For this review, take the finished solid that the model builds, in its own axes (mm). Face numbers are marked on the shaded views. A direction names the side the tool comes from. Round coordinates to 2 decimals unless told otherwise and drop trailing zeros. Order: outer loops, then holes, each group sorted by start corner. A loop starts at its lowest first (then second) coordinate and runs counter-clockwise, first axis right, second up. Notation, with made-up numbers: M 34.25,79 L 48.25,79 A19 ccw 48.25,98 Z; hole C -7.5,12.25 d4. An arc over 180 degrees is marked long. Answer as a JSON object with one key per item and string values.
Autodesk Inventor part; units mm, degrees
ref_plane "bolt_XY" through (0, 0, 0) normal (1, 0, 0) x (0, 0, -1)
ref_plane "bolt_YZ" through (0, 0, 0) normal (0, 0, -1) x (0, 1, 0)
ref_plane "bolt_ZX" through (0, 0, 0) normal (0, 1, 0) x (1, 0, 0)
sketch "Sketch_1" plane through (0, 0, 0) normal (0, 0, 1) x (1, 0, 0)
  line L0 (10, 0) -> (-5, 0)
  line L1 (-5, 0) -> (-5, 4.25)
  line L2 (-5, 4.25) -> (0, 4.25)
  line L3 (0, 4.25) -> (0, 2.5)
  line L4 (0, 2.5) -> (9.5095, 2.5)
  line L5 (9.5095, 2.5) -> (10, 2.0095)
  line L6 (10, 2.0095) -> (10, 0)
  line L7 (10, 0) -> (-5, 0)
revolve "Revolution1" add sketch "Sketch_1" angle 360 about axis through (10, 0, 0) along (1, 0, 0)
thread "Thread1"
sketch "Sketch_4" plane through (0, 0, 0) normal (0, 0, 1) x (1, 0, 0)
  line L0 (-1.9641, 0) -> (-5, 0)
  line L1 (-5, 0) -> (-5, 2)
  line L2 (-5, 2) -> (-2.5, 2)
  line L3 (-2.5, 2) -> (-1.9641, 0)
  line L4 (-1.9641, 0) -> (-5, 0)
revolve "Revolution2" cut sketch "Sketch_4" angle 360 about axis through (-1.9641, 0, 0) along (1, 0, 0)
sketch "Sketch_3" plane through (-5, 0, 0) normal (1, 0, 0) x (0, 0, -1)
  line L0 (-2, 1.1547) -> (-2, -1.1547)
  line L1 (-2, -1.1547) -> (0, -2.3094)
  line L2 (0, -2.3094) -> (2, -1.1547)
  line L3 (2, -1.1547) -> (2, 1.1547)
  line L4 (2, 1.1547) -> (0, 2.3094)
  line L5 (0, 2.3094) -> (-2, 1.1547)
extrude "Extrusion1" cut sketch "Sketch_3" along normal blind 2.5
ref_plane "bolt_XY" through (0, 0, 0) normal (1, 0, 0) x (0, 0, -1)
ref_plane "bolt_YZ" through (0, 0, 0) normal (0, 0, -1) x (0, 1, 0)
ref_plane "bolt_ZX" through (0, 0, 0) normal (0, 1, 0) x (1, 0, 0)
ref_plane "nut_XY" through (10, 0, 0) normal (1, 0, 0) x (0, 0, -1)
ref_plane "nut_YZ" through (10, 0, 0) normal (0, 0, -1) x (0, 1, 0)
ref_plane "nut_ZX" through (10, 0, 0) normal (0, 1, 0) x (1, 0, 0)
properties part number "CBM5-10" material "MISUMI"
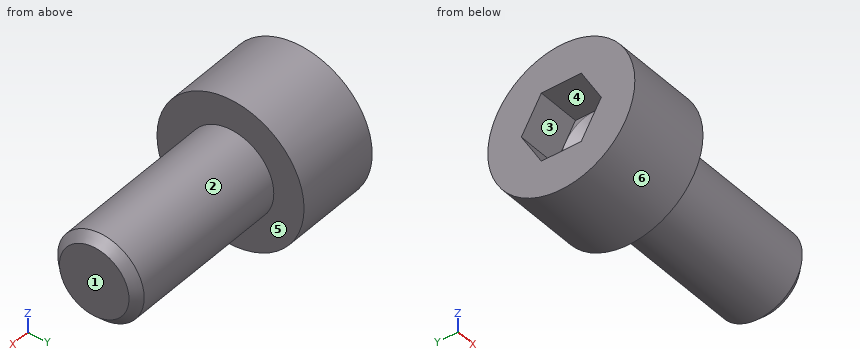
1) Add section C-C on x = 1.5. State the section outline as (y, z) points, and give its area (3 significant figures).
Geometry check:
{"outline": "C 0,0 d5", "area": "19.6 mm²"}
2) Add section A-A on x = -1.75. State the section outline as (y, z) points.
Geometry check:
{"outline": "C 0,0 d8.5"}
3) Machinability: for the marked faces 1, 2 and 3, which of the approach directions +Z, -Z, +X, -X, +Y, -Y give a long, thin tool a straight path to every point of the face, cutting with its end or side? Answer none if there is none.
Geometry check:
{"face 1": "+Z, -Z, +X, +Y, -Y", "face 2": "+X", "face 3": "-X"}
4) Mouldability with a two-part tool opening along Y and no side actions: class the marked faces 4, 5 and 6 as +Y half, -Y half, draft (parallel to the pull), parting line (faces both ways), or undercut.
Geometry check:
{"face 4": "undercut", "face 5": "draft", "face 6": "parting line"}
5) For L1, parallel to X at y = 2.75, z = -1.25; L2, parallel to Y at x = -0.25, z = -3.75; L3, parallel to Z at x = -2.75, y = 0.75, list the stretches that pass through material, from the lowest coordinate up.
Geometry check:
{"L1": "x = -5 to 0", "L2": "y = -2 to 2", "L3": "z = -4.18 to -2, 2 to 4.18"}
6) Insertion check: P1, Ø1.5, axis at x = -1, y = -1.5, coming from the +Z side; P2, Ø3, axis at x = 6, y = -1.5, coming from the +Z side; P3, Ø2, axis at x = 6, z = 1.5, coming from the +Y side; P4, Ø5, axis at y = 3, z = 2, coming from the +X side. Each pin has a flat end and moves straight along its axis. Give the tip position at first contact, or say it passes through.
Geometry check:
{"P1": "stops at z = 4.18", "P2": "stops at z = 2.5", "P3": "stops at y = 2.45", "P4": "stops at x = 10"}
7) Add section B-B on y = 3. State the section outline as (x, z) points, and give its area (3 significant figures).
Geometry check:
{"outline": "M -5,-3.01 L 0,-3.01 L 0,3.01 L -5,3.01 Z", "area": "30.1 mm²"}
